from build123d import *

# Parameters (mm, degrees)
SKETCH1_R           = 4.826
BOSS_EXTRUDE1_DEPTH = 50


with BuildPart() as part:
    # Sketch1 → Boss-Extrude1 (new body)
    with BuildSketch(Plane.XY):
        with BuildLine():
            Line((-20, 120.65), (-28.89, 120.65))
            Line((-28.89, 120.65), (-28.89, 102.65))
            Line((-28.89, 102.65), (-37.89, 102.65))
            Line((-37.89, 102.65), (-37.89, 126.65))
            ThreePointArc((-37.89, 126.65), (-36.718427125, 129.478427125), (-33.89, 130.65))
            Line((-33.89, 130.65), (-9.68, 130.65))
            ThreePointArc((-9.68, 130.65), (-2.608932188, 127.721067812), (0.32, 120.65))
            Line((0.32, 120.65), (0.32, 28.169089442))
            ThreePointArc((0.32, 28.169089442), (2.122439387, 22.441961017), (6.88, 18.779392961))
            ThreePointArc((6.88, 18.779392961), (11.454256851, -16.395121226), (-20, 0))
            Line((-20, 0), (-20, 120.65))
        make_face()
        Circle(SKETCH1_R, mode=Mode.SUBTRACT)
    extrude(amount=BOSS_EXTRUDE1_DEPTH)


solid = part.part
Input: part model. Units: mm. Frame: model coordinates. A direction names the side the tool comes from. Coordinates: 2 decimals unless noted, no trailing zeros. Loops run counter-clockwise (first coordinate to the right, second up) from the corner with the lowest first, then second, coordinate; pieces in that order, holes last. Notation, with made-up numbers: (-0.5, -36) -> (53.5, -36) arc R12 ccw to (53.5, -29) -> close; hole circle Ø8 at (58.25, -25). An arc over 180 degrees is marked (long way). Write each question's results on one line, items separated by ' | '. Start each with the question number.
Q1. Reachability of faces 1 (the flat face through (-24, 120.65, 25)), 2 (the flat face through (-33, 102.65, 25)), 3 (the cylindrical face through (-36.749, 129.447, 24.65)), 4 (the flat face through (0.32, 75, 25)), 5 (the flat face through (-22, 130.65, 25)) from +Z, -Z, +X, -X, +Y, -Y: full face, straight path, thin tool, end or side. Return the list, or none.
Q2. Pull-direction query (X, two-part tool) for faces 6 (the flat face through (-37.89, 114, 25)), 7 (the cylindrical face through (12, -16, 25)), 8 (the flat face through (-28.89, 112, 25)); classes: released by +X, released by -X, zero draft, split by the parting line, or undercut.
Q3. Section A-A, the plane z = 38.5. Return the cut outline in (x, y).
Q4. Ray query, line 1 (X direction, y = 46, z = 4); line 2 (Y direction, x = 2, z = 41); line 3 (X direction, y = 118, z = 29.5). Return the intervals inside material, ascending. Write a range as from..to.
Q5. Section C-C, the plane y = 21.5. Return the cut outline in (x, z), plus the area to 3 significant figures.
Q6. Section B-B, the plane x = 15. Return the cut outline in (y, z), plus the area to 3 significant figures.
Q7. Pin query (flat end, axial travel): pin 1 (6 mm diameter, centred on x = -10, z = 22, fed in from -Y) (3 decimals); pin 2 (9 mm diameter, centred on y = 108.5, z = 26.5, fed in from +X); pin 3 (7.5 mm diameter, centred on x = 0, y = 0, fed in from +Z); pin 4 (4.5 mm diameter, centred on x = -25.5, z = 21, fed in from -Y). Return the tip coordinate at first contact, or that it passes through.
Found:
1) face 1: +Z, -Z, -Y | face 2: +Z, -Z, -X, -Y | face 3: +Z, -Z, -X, +Y | face 4: +Z, -Z, +X, +Y | face 5: +Z, -Z, +X, -X, +Y
2) face 6: released by -X | face 7: split by the parting line | face 8: undercut
3) outline: (-37.89, 102.65) -> (-28.89, 102.65) -> (-28.89, 120.65) -> (-20, 120.65) -> (-20, 0) arc R20 ccw (long way) to (6.88, 18.78) arc R10 cw to (0.32, 28.17) -> (0.32, 120.65) arc R10 ccw to (-9.68, 130.65) -> (-33.89, 130.65) arc R4 ccw to (-37.89, 126.65) -> close; hole circle Ø9.65 at (0, 0)
4) line 1: -20..0.32 | line 2: -19.9..-4.39, 4.39..22.62 | line 3: -37.89..-28.89, -20..0.32
5) outline: (-20, 0) -> (2.87, 0) -> (2.87, 50) -> (-20, 50) -> close | area: 1,140 mm2
6) outline: (-13.23, 0) -> (13.23, 0) -> (13.23, 50) -> (-13.23, 50) -> close | area: 1,320 mm2
7) pin 1: y = -18.735 | pin 2: x = 0.32 | pin 3: through | pin 4: y = 120.65
